from build123d import *

# Parameters (mm, degrees)
SKETCH1_R                = 10
BOSS_EXTRUDE1_DEPTH      = 60
SKETCH2_R                = 3
BOSS_EXTRUDE2_DEPTH      = 23.645
BOSS_EXTRUDE3_DEPTH      = 9
BOSS_EXTRUDE3_DEPTH_BACK = 69
SKETCH3_R                = 3


with BuildPart() as part:
    # Sketch1 → Boss-Extrude1 (new body)
    with BuildSketch(Plane.XY):
        Circle(SKETCH1_R)
    extrude(amount=BOSS_EXTRUDE1_DEPTH)

    # Sketch2 → Boss-Extrude2 (add, symmetric)
    with BuildSketch(Plane(origin=(0, 0, 0), x_dir=(0, 0, -1), z_dir=(1, 0, 0))):
        with Locations((-30, 0)):
            Circle(SKETCH2_R)
    extrude(amount=BOSS_EXTRUDE2_DEPTH, both=True)

    # Sketch3 → Boss-Extrude3 (add, two sides: drawn at the far end of the back side and taken through both)
    with BuildSketch(Plane.XY.offset(60).offset(-BOSS_EXTRUDE3_DEPTH_BACK)):
        Circle(SKETCH3_R)
    extrude(amount=BOSS_EXTRUDE3_DEPTH + BOSS_EXTRUDE3_DEPTH_BACK)


solid = part.part
Read the model definition and answer for the solid it produces. Units are mm, in the model's axes. A direction names the side the tool comes from. Coordinates: 2 decimals unless noted, no trailing zeros. Loops run counter-clockwise (first coordinate to the right, second up) from the corner with the lowest first, then second, coordinate; pieces in that order, holes last. Notation, with made-up numbers: (15.25, 70.5) -> (45.25, 70.5) arc R9 cw to (45.25, 80.5) -> close; hole circle Ø4 at (-15.75, 78). An arc over 180 degrees is marked (long way). Write item = value, one per line. Start each with the question number.
1) The part is cut by section C-C, the plane y = 0. Determine the outline of the cut face in (x, z) (3 decimals), plus the area to 3 significant figures.
2) For faces 1 (the face through (17, 0, 33)), 2 (the face through (-16, 0, 33)), 3 (the face through (2.1, 2.4, 60)), determine the directions among +Z, -Z, +X, -X, +Y, -Y from which every point of the face is accessible in a straight line to the end or side of a thin tool.
3) The mould has two halves that part along Y. Classify faces 4 (the face through (-3, 0, 64)), 5 (the face through (2.1, 2.4, 0)): pulls with the +Y half, pulls with the -Y half, needs draft (parallel to the pull), parting line crosses it, or undercut.
4) Given P1, Ø10, axis at y = 1.5, z = 0, coming from the -X side; P2, Ø1, axis at x = 14.5, y = 0.5, coming from the -Z side; P3, Ø3, axis at x = -19, y = 0, coming from the +Z side, each flat-ended and moving along its own axis, determine where each tip first touches the part or whether it passes through.
5) The part is cut by section A-A, the plane x = 0. Determine the outline of the cut face in (y, z), plus the area to 3 significant figures.
6) The part is cut by section D-D, the plane z = 5. Determine the outline of the cut face in (x, y), plus the area to 3 significant figures.
7) The part is cut by section B-B, the plane z = 30. Determine the outline of the cut face in (x, y) (3 decimals), plus the area to 3 significant figures.
8) Find the intervals of material crossed by L1, parallel to Z at x = 2.5, y = -5.75; L2, parallel to Y at x = 3, z = 24.5; L3, parallel to X at y = -0.5, z = 8.5, in increasing order. Write a range as from..to.
Result:
q1.outline = (-23.645, 27) -> (-10, 27) -> (-10, 0) -> (-3, 0) -> (-3, -9) -> (3, -9) -> (3, 0) -> (10, 0) -> (10, 27) -> (23.645, 27) -> (23.645, 33) -> (10, 33) -> (10, 60) -> (3, 60) -> (3, 69) -> (-3, 69) -> (-3, 60) -> (-10, 60) -> (-10, 33) -> (-23.645, 33) -> close
q1.area = 1,470 mm²
q2.face_1 = +X
q2.face_2 = -X
q2.face_3 = +Z
q3.face_4 = parting line crosses it
q3.face_5 = needs draft
q4.P1 = -10
q4.P2 = 27
q4.P3 = 33
q5.outline = (-10, 0) -> (-3, 0) -> (-3, -9) -> (3, -9) -> (3, 0) -> (10, 0) -> (10, 60) -> (3, 60) -> (3, 69) -> (-3, 69) -> (-3, 60) -> (-10, 60) -> close
q5.area = 1,310 mm²
q6.outline = circle Ø20 at (0, 0)
q6.area = 314 mm²
q7.outline = (-23.645, -3) -> (-9.539, -3) arc R10 ccw to (9.539, -3) -> (23.645, -3) -> (23.645, 3) -> (9.539, 3) arc R10 ccw to (-9.539, 3) -> (-23.645, 3) -> close
q7.area = 480 mm²
q8.L1 = 0..60
q8.L2 = -9.54..9.54
q8.L3 = -9.99..9.99
